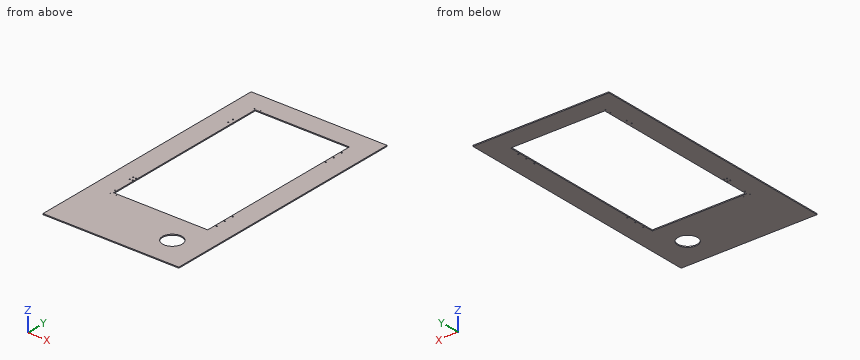
from build123d import *

# Parameters (mm, degrees)
SKETCH1_W           = 879.7036
SKETCH1_H           = 1641.475
BOSS_EXTRUDE1_DEPTH = 6.35
FILLET1_R           = 0.254
SKETCH2_W           = 609.6
SKETCH2_H           = 1117.6
CUT_EXTRUDE1_DEPTH  = 1863.353060507
SKETCH3_R           = 3.81
CUT_EXTRUDE2_DEPTH  = 1863.353060507
SKETCH5_R           = 63.5
CUT_EXTRUDE4_DEPTH  = 1863.353060507
SKETCH6_R           = 2.7
CUT_EXTRUDE5_DEPTH  = 1863.353060507


with BuildPart() as part:
    # Sketch1 → Boss-Extrude1 (new body)
    with BuildSketch(Plane.XY):
        with Locations((439.8518, -820.7375)):
            Rectangle(SKETCH1_W, SKETCH1_H)
    extrude(amount=BOSS_EXTRUDE1_DEPTH)

    # Fillet1
    fillet1_edges = [part.edges().sort_by_distance(p)[0] for p in [
        (879.7036, -1641.475, 3.175),
        (0, -1641.475, 3.175),
        (0, 0, 3.175),
        (879.7036, 0, 3.175),
    ]]
    fillet(fillet1_edges, radius=FILLET1_R)

    # Sketch2 → Cut-Extrude1 (cut, through all)
    with BuildSketch(Plane.XY.offset(6.35)):
        with Locations((439.8518, -691.134)):
            Rectangle(SKETCH2_W, SKETCH2_H)
    extrude(amount=-CUT_EXTRUDE1_DEPTH, mode=Mode.SUBTRACT)

    # Sketch3 → Cut-Extrude2 (cut, through all)
    with BuildSketch(Plane.XY.offset(6.35)):
        with Locations((754.3546, -204.724)):
            Circle(SKETCH3_R)
        with Locations((754.3546, -268.224)):
            Circle(SKETCH3_R)
        with Locations((754.3546, -331.724)):
            Circle(SKETCH3_R)
        with Locations((754.3546, -1190.244)):
            Circle(SKETCH3_R)
        with Locations((754.3546, -1126.744)):
            Circle(SKETCH3_R)
        with Locations((754.3546, -1063.244)):
            Circle(SKETCH3_R)
        with Locations((109.383049966, -1063.863000196)):
            Circle(SKETCH3_R)
        with Locations((127.383050034, -1063.863000196)):
            Circle(SKETCH3_R)
        with Locations((127.383050034, -1089.863000266)):
            Circle(SKETCH3_R)
        with Locations((109.383049966, -1089.863000266)):
            Circle(SKETCH3_R)
        with Locations((113.748448168, -280.289)):
            Circle(SKETCH3_R)
        with Locations((113.748448168, -318.389)):
            Circle(SKETCH3_R)
    extrude(amount=-CUT_EXTRUDE2_DEPTH, mode=Mode.SUBTRACT)

    # Sketch5 → Cut-Extrude4 (cut, through all)
    with BuildSketch(Plane.XY.offset(6.35)):
        with Locations((676.5036, -1445.7045)):
            Circle(SKETCH5_R)
    extrude(amount=-CUT_EXTRUDE4_DEPTH, mode=Mode.SUBTRACT)

    # Sketch6 → Cut-Extrude5 (cut, through all)
    with BuildSketch(Plane(origin=(0, 0, 0), x_dir=(-1, 0, 0), z_dir=(0, 0, -1))):
        with Locations(Location((-124.3, -1223.551, 0), (0, 0, 90))):
            Circle(SKETCH6_R)
        with Locations(Location((-124.3, -1263.175, 0), (0, 0, 90))):
            Circle(SKETCH6_R)
        with Locations(Location((-163.924, -1263.175, 0), (0, 0, 90))):
            Circle(SKETCH6_R)
        with Locations(Location((-163.924, -124.3, 0), (0, 0, 270))):
            Circle(SKETCH6_R)
        with Locations(Location((-124.3, -124.3, 0), (0, 0, 270))):
            Circle(SKETCH6_R)
        with Locations(Location((-124.3, -163.924, 0), (0, 0, 270))):
            Circle(SKETCH6_R)
    extrude(amount=-CUT_EXTRUDE5_DEPTH, mode=Mode.SUBTRACT)


solid = part.part
Can you work these out from the model? Positions are in its coordinate system, mm. Coordinates: 2 decimals unless noted, no trailing zeros. Loops run counter-clockwise (first coordinate to the right, second up) from the corner with the lowest first, then second, coordinate; pieces in that order, holes last. Notation, with made-up numbers: M -25.5,24 L 26.5,24 A13 ccw 26.5,37 Z; hole C -3.5,-25.75 d7. An arc over 180 degrees is marked long. Answer as CSV lines item,"result". Start each with the question number.
1. Suppose I cut it at A-A, the plane x = 296.5. List the corners of the cut face in (y, z) for me (3 decimals).
2. If I drill on probe 1 along X at (y, z) = (-124.3, 1.75); probe 2 along Y at (x, z) = (679, 4.5) (3 decimals); probe 3 along Y at (x, z) = (439.5, 1.5) (3 decimals), over which ranges is the centre line in solid material (lowest first)? Write a range as [from, to].
3. Suppose I cut it at C-C, the plane z = 4.25. Count the separate pieces of the cut face and the enclosed holes in it, plus the area to 3 significant figures.
4. For pin 1 Ø12 at (x, y) = (754.35, -331.72) entering from +Z, with a flat end and sliding along its axis, tell me the tip position at first contact or that it passes through.
5. Suppose I cut it at D-D, the plane x = 688. List the corners of the cut face in (y, z) for me (3 decimals).
6. Suppose I cut it at B-B, the plane y = -648.5. List the corners of the cut face in (x, z) for me, plus the area to 3 significant figures.
Output:
1,outline,"M -1641.475,0 L -1249.934,0 L -1249.934,6.35 L -1641.475,6.35 Z; M -132.334,0 L 0,0 L 0,6.35 L -132.334,6.35 Z"
2,probe 1,"x = [0, 121.6], [127, 161.22], [166.62, 879.7]"
2,probe 2,"y = [-1641.475, -1509.155], [-1382.254, -1249.934], [-132.334, 0]"
2,probe 3,"y = [-1641.475, -1249.934], [-132.334, 0]"
3,separate pieces,"1"
3,enclosed holes,"20"
3,area,"749,000 mm^2"
4,pin 1,"stops at z = 6.35"
5,outline,"M -1641.475,0 L -1508.155,0 L -1508.155,6.35 L -1641.475,6.35 Z; M -1383.254,0 L -1249.934,0 L -1249.934,6.35 L -1383.254,6.35 Z; M -132.334,0 L 0,0 L 0,6.35 L -132.334,6.35 Z"
6,outline,"M 0,0 L 135.05,0 L 135.05,6.35 L 0,6.35 Z; M 744.65,0 L 879.7,0 L 879.7,6.35 L 744.65,6.35 Z"
6,area,"1,720 mm^2"
